```python
from build123d import *

# Parameters (mm, degrees)
SCHIZZO1_R                    = 17.5
ESTRUSIONE_ESTRUSIONE1_DEPTH  = 50
TAGLIO_ESTRUSIONE1_REACH      = 144.171
SCHIZZO10_R                   = 16.3
TAGLIO_ESTRUSIONE3_DEPTH      = 143.170672106
TAGLIO_ESTRUSIONE3_DEPTH_BACK = 143.170672106
SCHIZZO14_R                   = 2.5
SKETCH1_R                     = 16.3
SKETCH1_R_2                   = 14.8
BOSS_EXTRUDE3_DEPTH           = 15
SKETCH2_R                     = 2.2
BOSS_EXTRUDE4_DEPTH           = 5
CUT_EXTRUDE1_DEPTH            = 146.365917733
CUT_EXTRUDE1_DEPTH_BACK       = 146.365917733
SKETCH4_R                     = 2.5
CUT_EXTRUDE2_DEPTH            = 146.365917738
CUT_EXTRUDE2_DEPTH_BACK       = 146.365917738
SKETCH5_R                     = 2.5


with BuildPart() as part:
    # Schizzo1 → Estrusione-Estrusione1 (new body)
    with BuildSketch(Plane(origin=(0, 0, 0), x_dir=(1, 0, 0), z_dir=(0, 1, 0))):
        with Locations(Location((0, 0, 0), (0, 0, 270))):
            Circle(SCHIZZO1_R)
    extrude(amount=ESTRUSIONE_ESTRUSIONE1_DEPTH)

    # Schizzo7 → Rivoluzione1 (revolve)
    with BuildSketch(Plane.XY):
        with BuildLine():
            Line((0, 140), (-2.55, 140))
            add(Edge.make_bspline(
                [(-2.55, 140), (-17.5, 113.62789219), (-17.5, 50)],
                knots=[0, 0, 0, 1, 1, 1], degree=2))
            Line((-17.5, 50), (-16.3, 50))
            add(Edge.make_bspline(
                [(-2, 138.8), (-16.3, 113.62789219), (-16.3, 50)],
                knots=[0, 0, 0, 1, 1, 1], degree=2))
            Line((-2, 138.8), (0, 138.8))
            Line((0, 138.8), (0, 140))
        make_face()
    revolve(axis=Axis((0, 50, 0), (0, 1, 0)))

    # Schizzo10 → Taglio-Estrusione1 (cut, up to next)
    with BuildSketch(Plane(origin=(0, 0, 0), x_dir=(1, 0, 0), z_dir=(0, 1, 0)), mode=Mode.PRIVATE) as taglio_estrusione1_sk1:
        with Locations(Location((0, 0, 0), (0, 0, 90))):
            Circle(SCHIZZO10_R)
    taglio_estrusione1_tool1 = extrude(taglio_estrusione1_sk1.sketch, amount=TAGLIO_ESTRUSIONE1_REACH, mode=Mode.PRIVATE) & part.part
    add(taglio_estrusione1_tool1.solids().sort_by_distance((0, 0, 0))[0], mode=Mode.SUBTRACT)

    # Schizzo14 → Taglio-Estrusione3 (cut, two sides: drawn at the far end of the back side and taken through both)
    with BuildSketch(Plane(origin=(0, 140, 0), x_dir=(1, 0, 0), z_dir=(0, 1, 0)).offset(-TAGLIO_ESTRUSIONE3_DEPTH_BACK)):
        with Locations(Location((0, 0, 0), (0, 0, 90))):
            Circle(SCHIZZO14_R)
    extrude(amount=TAGLIO_ESTRUSIONE3_DEPTH + TAGLIO_ESTRUSIONE3_DEPTH_BACK, mode=Mode.SUBTRACT)

    # Sketch1 → Boss-Extrude3 (add)
    with BuildSketch(Plane.XZ):
        with Locations(Location((0, 0, 0), (0, 0, 270))):
            Circle(SKETCH1_R)
        with Locations(Location((0, 0, 0), (0, 0, 270))):
            Circle(SKETCH1_R_2, mode=Mode.SUBTRACT)
    extrude(amount=-BOSS_EXTRUDE3_DEPTH)

    # Sketch2 → Boss-Extrude4 (add)
    # profile 1 of 2: a face of its own
    with BuildSketch(Plane.XZ):
        with BuildLine():
            ThreePointArc((8.3, 4.3829214), (3.9170786, 0), (8.3, -4.3829214))
            Line((8.3, -4.3829214), (14.136123938, -4.3829214))
            ThreePointArc((14.136123938, -4.3829214), (14.8, 0), (14.136123938, 4.3829214))
            Line((14.136123938, 4.3829214), (8.3, 4.3829214))
        make_face()
        with Locations(Location((8.3, 0, 0), (0, 0, 270))):
            Circle(SKETCH2_R, mode=Mode.SUBTRACT)
    # profile 2 of 2: a face of its own
    with BuildSketch(Plane.XZ):
        with BuildLine():
            Line((-8.3, 4.3829214), (-14.136123938, 4.3829214))
            ThreePointArc((-14.136123938, 4.3829214), (-14.8, 0), (-14.136123938, -4.3829214))
            Line((-14.136123938, -4.3829214), (-8.3, -4.3829214))
            ThreePointArc((-8.3, -4.3829214), (-3.9170786, 0), (-8.3, 4.3829214))
        make_face()
        with Locations(Location((-8.3, 0, 0), (0, 0, 270))):
            Circle(SKETCH2_R, mode=Mode.SUBTRACT)
    extrude(amount=-BOSS_EXTRUDE4_DEPTH)

    # Sketch4 → Cut-Extrude1 (cut, two sides: drawn at the far end of the back side and taken through both)
    with BuildSketch(Plane.XY.offset(17.5).offset(-CUT_EXTRUDE1_DEPTH_BACK)):
        with Locations((0, 35)):
            Circle(SKETCH4_R)
    extrude(amount=CUT_EXTRUDE1_DEPTH + CUT_EXTRUDE1_DEPTH_BACK, mode=Mode.SUBTRACT)

    # Sketch5 → Cut-Extrude2 (cut, two sides: drawn at the far end of the back side and taken through both)
    with BuildSketch(Plane(origin=(17.5, 0, 0), x_dir=(0, 0, -1), z_dir=(1, 0, 0)).offset(-CUT_EXTRUDE2_DEPTH_BACK)):
        with Locations((0, 35)):
            Circle(SKETCH5_R)
    extrude(amount=CUT_EXTRUDE2_DEPTH + CUT_EXTRUDE2_DEPTH_BACK, mode=Mode.SUBTRACT)


solid = part.part
```
The model under review builds one solid part; all positions refer to its coordinate system, in mm. A direction names the side the tool comes from. Round coordinates to 2 decimals unless told otherwise and drop trailing zeros. Loops run counter-clockwise (first coordinate to the right, second up) from the corner with the lowest first, then second, coordinate; pieces in that order, holes last.
1) Consider section C-C on y = 39. State the section outline as (x, z) points.
Values follow:
outline: circle Ø35 at (0, 0); hole circle Ø32.6 at (0, 0)
2) The part is to be moulded in two halves that separate along X. For faces 4 (the face through (16.794, 35.751, -2.385)), 5 (the face through (-15.526, 24.65, 8.075)), 6 (the face through (-11, 2, -4.383)), say which applies: pulls with the +X half, pulls with the -X half, needs draft (parallel to the pull), parting line crosses it, or undercut.
Values follow:
face 4: needs draft
face 5: parting line crosses it
face 6: undercut
3) Wall thickness on line 1 along X through (y, z) = (2.9, 0); line 2 along Z through (x, y) = (0, 12); line 3 along X through (y, z) = (29, -3.5): over which ranges is each line inside the solid? List them lowest first.
Values follow:
line 1: x = -17.5 to -10.5, -6.1 to -3.92, 3.92 to 6.1, 10.5 to 17.5
line 2: z = -17.5 to -14.8, 14.8 to 17.5
line 3: x = -17.15 to -15.92, 15.92 to 17.15
4) Clearance check with flat-ended pins moving along their axes: P1, Ø1.5, axis at x = 12.5, y = 3, coming from the -Z side; P2, Ø4, axis at x = 0, y = 35, coming from the +Z side; P3, Ø5.5, axis at x = -11.5, y = 2.5, coming from the +Z side; P4, Ø2, axis at y = 95.5, z = 9, coming from the -X side. State where each tip first meets the part, or that it passes through.
Values follow:
P1: stops at z = -12.97
P2: passes through
P3: stops at z = 15.16
P4: stops at x = -12.75
5) Tool access review of faces 1 (the face through (-11, 2, 4.383)), 2 (the face through (2.44, 138.94, 0.54)), 3 (the face through (-5.67, 7.4, -13.67)): name each direction out of +Z, -Z, +X, -X, +Y, -Y from which nothing blocks a thin tool from reaching the whole face with its end or side.
Values follow:
face 1: -Y
face 2: +Y, -Y
face 3: none
6) Consider section A-A on x = 0. Give the number of separate pieces and of enclosed holes in the cut face, then the cut area to 3 significant figures.
Values follow:
separate pieces: 4
enclosed holes: 0
area: 354 mm2
